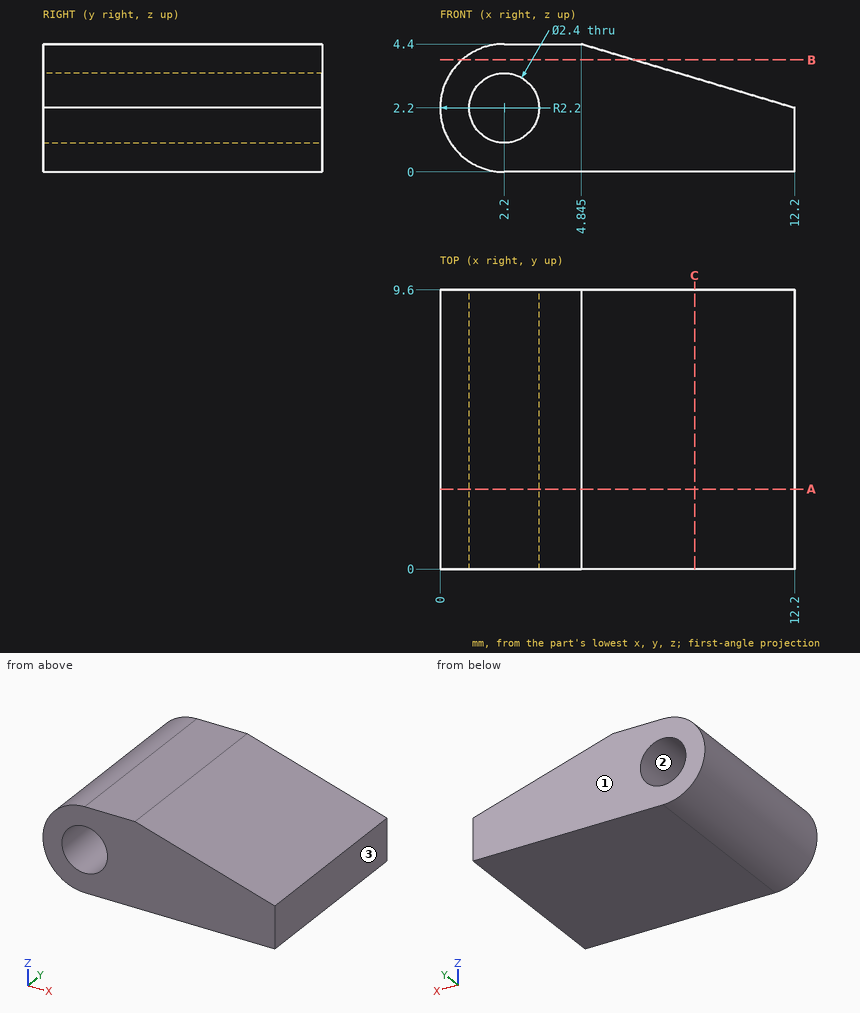
Input: dimensioned drawing with shaded views. Units: mm. Origin: part minimum x, y, z. Round coordinates to 2 decimals unless told otherwise and drop trailing zeros. Order: outer loops, then holes, each group sorted by start corner. A loop starts at its lowest first (then second) coordinate and runs counter-clockwise, first axis right, second up. Notation, with made-up numbers: (86, 56.25) -> (136, 56.25) arc R34 ccw to (136, 94.25) -> close; hole circle Ø8 at (32.5, 59.25). An arc over 180 degrees is marked (long way). Put each result on its own line as item: value. Start each with the question number.
Q1. Line query: probe 1 along X at (y, z) = (4, 2); probe 2 along Z at (x, y) = (2, 4); probe 3 along X at (y, z) = (1, 1.25) (1 decimal). Output: solid intervals per line, ascending.
Q2. Pull-direction query (X, two-part tool) for the marked faces 1, 2 and 3; classes: +X half, -X half, draft (parallel to the pull), parting line (faces both ways), or undercut.
Q3. Section A-A on y = 2.75. Return the cut outline in (x, z) (1 decimal), and give its area (3 significant figures).
Q4. Section B-B on z = 3.85. Return the cut outline in (x, y) (1 decimal).
Q5. Section C-C on x = 8.75. Return the cut outline in (y, z), and give its area (3 significant figures).
Ans:
1. probe 1: x = 0.01 to 1.02, 3.38 to 12.2
1. probe 2: z = 0.01 to 1.02, 3.38 to 4.39
1. probe 3: x = 0.2 to 1.5, 2.9 to 12.2
2. face 1: draft
2. face 2: undercut
2. face 3: +X half
3. outline: (2.2, 0) -> (12.2, 0) -> (12.2, 2.2) -> (4.8, 4.4) -> (2.2, 4.4) arc R2.2 ccw to start; hole circle Ø2.4 at (2.2, 2.2)
3. area: 39.0 mm2
4. outline: (0.7, 0) -> (6.7, 0) -> (6.7, 9.6) -> (0.7, 9.6) -> close
5. outline: (0, 0) -> (9.6, 0) -> (9.6, 3.23) -> (0, 3.23) -> close
5. area: 31.0 mm2
